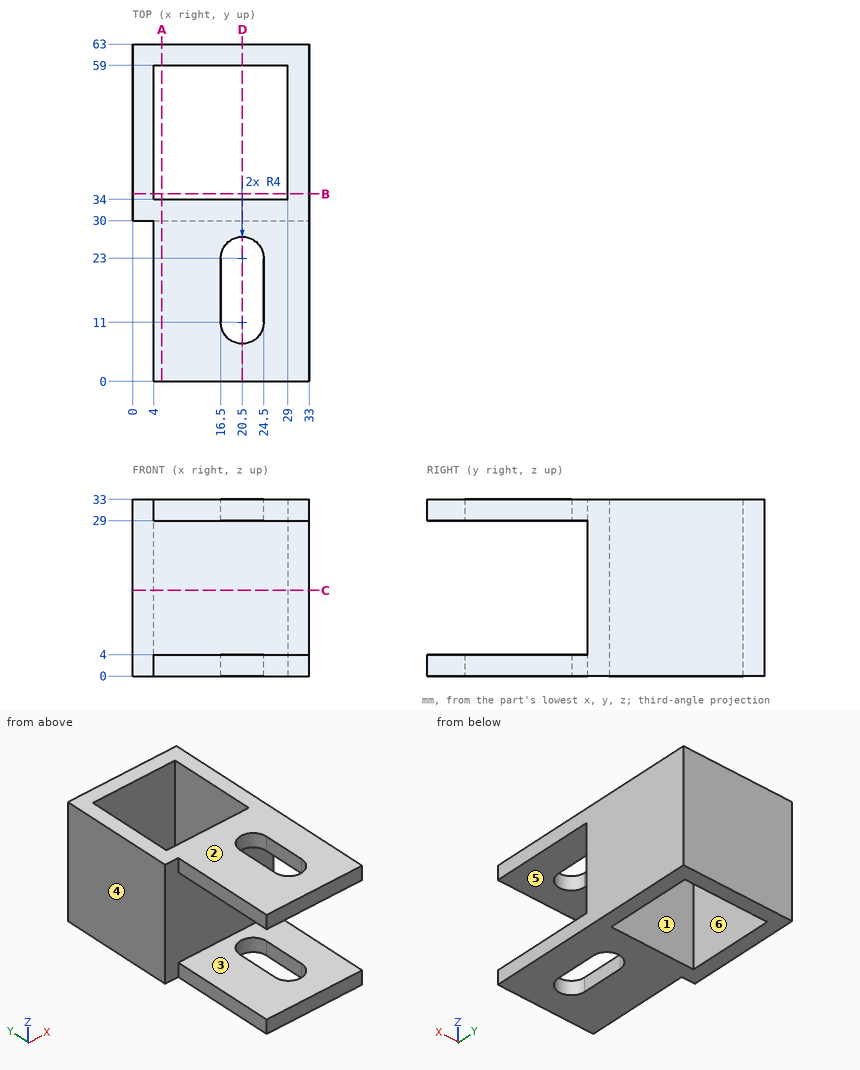
Part print with two shaded views. Sizes in mm from the minimum x, y, z corner. A direction names the side the tool comes from. Round coordinates to 2 decimals unless told otherwise and drop trailing zeros. Loops run counter-clockwise (first coordinate to the right, second up) from the corner with the lowest first, then second, coordinate; pieces in that order, holes last.
Item 1: Saw through at D-D (x = 20.5). List the corners of the cut face in (y, z), then the cut area to 3 significant figures.
Item 2: Drill centre lines: line 1 along Z through (x, y) = (8.5, 6); line 2 along Y through (x, z) = (7.5, 3); line 3 along Y through (x, z) = (21, 11). Where is each one in solid material? Low to high.
Item 3: Pin check, flat tips, straight feed: P1, Ø12, axis at x = 26.5, z = 27, coming from the -Y side; P2, Ø4.5, axis at y = 19.5, z = 2.5, coming from the -X side; P3, Ø12.5, axis at x = 15.5, z = 22, coming from the -Y side. Stop position of each tip, or through.
Item 4: Two-plate mould, pull along X, no slides. Class the marked faces 4, 5 and 6: released by +X, released by -X, zero draft, split by the parting line, or undercut.
Item 5: Saw through at A-A (x = 5.5). List the corners of the cut face in (y, z), then the cut area to 3 significant figures.
Item 6: Saw through at B-B (y = 35). List the corners of the cut face in (x, z), then the cut area to 3 significant figures.
Item 7: Saw through at C-C (z = 16). List the corners of the cut face in (x, y), then the cut area to 3 significant figures.
Item 8: Which spindle directions (+Z, -Z, +X, -X, +Y, -Y) get a long thin tool onto all of the face, cutting with end or side? Do the marked faces 1, 2 and 3. Say none if no direction does.
Worked answers:
1. outline: (0, 0) - (7, 0) - (7, 4) - (0, 4) - close; (0, 29) - (7, 29) - (7, 33) - (0, 33) - close; (27, 0) - (34, 0) - (34, 33) - (27, 33) - (27, 29) - (30, 29) - (30, 4) - (27, 4) - close; (59, 0) - (63, 0) - (63, 33) - (59, 33) - close
1. area: 344 mm2
2. line 1: z = 0 to 4, 29 to 33
2. line 2: y = 0 to 34, 59 to 63
2. line 3: y = 30 to 34, 59 to 63
3. P1: stops at y = 0
3. P2: stops at x = 4
3. P3: stops at y = 30
4. face 4: released by -X
4. face 5: zero draft
4. face 6: undercut
5. outline: (0, 0) - (34, 0) - (34, 33) - (0, 33) - (0, 29) - (30, 29) - (30, 4) - (0, 4) - close; (59, 0) - (63, 0) - (63, 33) - (59, 33) - close
5. area: 504 mm2
6. outline: (0, 0) - (4, 0) - (4, 33) - (0, 33) - close; (29, 0) - (33, 0) - (33, 33) - (29, 33) - close
6. area: 264 mm2
7. outline: (0, 30) - (33, 30) - (33, 63) - (0, 63) - close; hole (4, 34) - (29, 34) - (29, 59) - (4, 59) - close
7. area: 464 mm2
8. face 1: +Z, -Z
8. face 2: +Z, +X, -X, +Y, -Y
8. face 3: +X, -X, -Y
